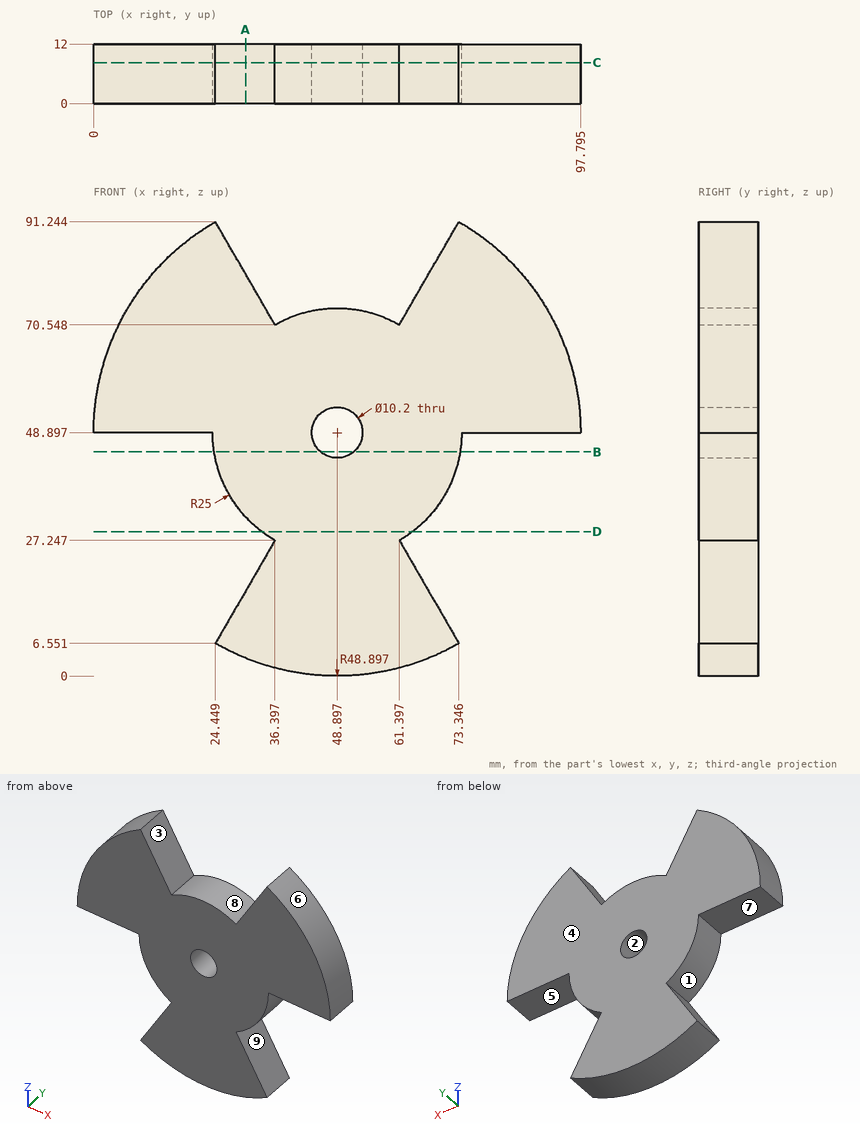
Verification items for this drawing (mm, ordinates from the low corner). A direction names the side the tool comes from. Coordinates: 2 decimals unless noted, no trailing zeros. Loops run counter-clockwise (first coordinate to the right, second up) from the corner with the lowest first, then second, coordinate; pieces in that order, holes last. Notation, with made-up numbers: (61.5, 14.25) - (69.5, 14.25) arc R5 ccw to (69.5, 18.25) - close; hole circle Ø4 at (-4.75, 62). An arc over 180 degrees is marked (long way). One line per item, written item: value. Start each with the question number.
(1) Depth check by flat-ended pin: P1, Ø2, axis at y = 8, z = 73.5, coming from the -X side; P2, Ø6, axis at x = 89, y = 3.5, coming from the -Z side; P3, Ø4, axis at y = 4.5, z = 58.5, coming from the +X side. Enter the tip coordinate at first touch or a pass-through.
(2) Cross-section at A-A on x = 30.5. Enter the section's corners in (y, z).
(3) Cross-section at D-D on z = 29. Enter the section's corners in (x, y), plus the area to 3 significant figures.
(4) Cross-section at B-B on z = 45. Enter the section's corners in (x, y).
(5) Cross-section at C-C on y = 8.25. Enter the section's corners in (x, z) (1 decimal), plus the area to 3 significant figures.
(6) Mould release check, pull along X, two halves, no side actions. Record for the marked faces 1, 2, 3 and 4: released by +X, released by -X, zero draft, split by the parting line, or undercut.
(7) Material ranges on line 1 (X direction, y = 4, z = 79) (1 decimal); line 2 (Z direction, x = 62.5, y = 9.75) (1 decimal); line 3 (X direction, y = 2.5, z = 81.5) (1 decimal), recorded low to high. Write a range as [from, to].
(8) Tool access check on the marked faces 5, 6, 7, 8 and 9. Record the directions out of +Z, -Z, +X, -X, +Y, -Y that give a thin tool (end or side, any length) a straight path to the whole face; none if there is none.
Results below:
1. P1: stops at x = 6.07
1. P2: stops at z = 48.9
1. P3: stops at x = 97.2
2. outline: (0, 3.59) - (12, 3.59) - (12, 17.03) - (0, 17.03) - close; (0, 31.97) - (12, 31.97) - (12, 80.76) - (0, 80.76) - close
3. outline: (33.76, 0) - (64.03, 0) - (64.03, 12) - (33.76, 12) - close
3. area: 363 mm2
4. outline: (24.2, 0) - (45.61, 0) - (45.61, 12) - (24.2, 12) - close; (52.19, 0) - (73.59, 0) - (73.59, 12) - (52.19, 12) - close
5. outline: (0, 48.9) - (23.9, 48.9) arc R25 ccw to (36.4, 27.2) - (24.4, 6.6) arc R48.9 ccw to (73.3, 6.6) - (61.4, 27.2) arc R25 ccw to (73.9, 48.9) - (97.8, 48.9) arc R48.9 ccw to (73.3, 91.2) - (61.4, 70.5) arc R25 ccw to (36.4, 70.5) - (24.4, 91.2) arc R48.9 ccw to start; hole circle Ø10.2 at (48.9, 48.9)
5. area: 4,660 mm2
6. face 1: released by -X
6. face 2: undercut
6. face 3: undercut
6. face 4: zero draft
7. line 1: x = [10.4, 31.5], [66.3, 87.4]
7. line 2: z = [1.9, 25.3], [27.9, 72.5]
7. line 3: x = [12.5, 30.1], [67.7, 85.3]
8. face 5: -Z, +X, +Y, -Y
8. face 6: +Z, +X, +Y, -Y
8. face 7: -Z, -X, +Y, -Y
8. face 8: +Z, +Y, -Y
8. face 9: +X, +Y, -Y
